Check sheet for the modelled part. Datum: model origin and axes. Units: mm. A direction names the side the tool comes from. Give positions to 0.01 mm unless a question says otherwise; leave off trailing zeros. Loops run counter-clockwise (first coordinate to the right, second up) from the corner with the lowest first, then second, coordinate; pieces in that order, holes last. Notation, with made-up numbers: (86, 84.25) -> (126, 84.25) arc R8 cw to (126, 88.25) -> close; hole circle Ø8 at (31.25, 35). An arc over 180 degrees is marked (long way). Write each question's results on one line, items separated by ' | '. Start each with the question number.
1. Cross-section at A-A on x = -12. Record the boundary of the cut face in (y, z).
2. Mould release check, pull along X, two halves, no side actions. Record for faces 6 (the face through (0, -23, 48)), 7 (the face through (60, -22.5, 24.2)), 8 (the face through (-17.969, -27.137, 46.028)): +X half, -X half, draft (parallel to the pull), parting line (faces both ways), or undercut.
3. Tool access check on faces 1 (the face through (-31, -25, 24)), 2 (the face through (-59.5, 0, 26)), 3 (the face through (26.13, 28.19, 26.38)), 4 (the face through (6, -26, 35)), 5 (the face through (-0.4, -32.5, 44)). Record the directions out of +Z, -Z, +X, -X, +Y, -Y that give a thin tool (end or side, any length) a straight path to the whole face; none if there is none.
4. Cross-section at D-D on x = 41.5. Record the boundary of the cut face in (y, z).
5. Gauge pin test, flat ends, axial feed: pin 1 Ø3.5 at (x, y) = (18, -29) entering from +Z; pin 2 Ø1 at (x, z) = (43, 15.5) entering from +Y; pin 3 Ø2.5 at (y, z) = (-27, 24.5) entering from -X; pin 4 Ø5 at (x, z) = (-28, 20) entering from -Y. Record the tip position at first contact, or that the pin passes through.
6. Material ranges on L1, parallel to Y at x = -17, z = 46; L2, parallel to Y at x = -46.5, z = 26; L3, parallel to X at y = -6, z = 38, recorded low to high. Write a range as from..to.
7. Cross-section at B-B on y = -8. Record the boundary of the cut face in (x, z), and give its area (3 significant figures).
8. Cross-section at C-C on x = 8.5. Record the boundary of the cut face in (y, z), and give its area (3 significant figures).
from build123d import *

# Parameters (mm, degrees)
SKETCH_1_W             = 125
SKETCH_1_H             = 50
EXTRUDE_1_DEPTH        = 3
SKETCH_2_W             = 125
SKETCH_2_H             = 50
SKETCH_2_W_2           = 119
SKETCH_2_H_2           = 44
EXTRUDE_2_DEPTH        = 45
EXTRUDE_START          = 33
EXTRUDE_3_DEPTH        = 12
SKETCH_6_W             = 50
SKETCH_6_H             = 8
SKETCH_6_R             = 2.1
EXTRUDE_7_DEPTH        = 4
FILLET_START           = 43
FILLET_10_DEPTH        = 5
FILLET_START_2         = 44
FILLET_10_2_DEPTH      = 4
CHAMFER_2_SIZE         = 6
FILLET_12_R            = 2
CHAMFER_3_SIZE         = 5
SKETCH_7_R             = 1.35
CUT_EXTRUDE_1_DEPTH    = 86.435648297
PATTERN_LINEAR_2_COUNT = 2
PATTERN_LINEAR_2_PITCH = 39
FILLET_13_R            = 2
SKETCH_8_W             = 12
SKETCH_8_H             = 8
CUT_EXTRUDE_2_DEPTH    = 86.435648297
FILLET_14_R            = 3
SKETCH_9_W             = 61.451933819
SKETCH_9_H             = 10.261376853
CUT_EXTRUDE_3_DEPTH    = 70
SKETCH_10_R            = 3
SKETCH_10_R_2          = 1.5
EXTRUDE_8_DEPTH        = 6.47


with BuildPart() as part:
    # 草图1 → 凸台-拉伸1 (new body)
    with BuildSketch(Plane.XY):
        Rectangle(SKETCH_1_W, SKETCH_1_H)
    extrude(amount=EXTRUDE_1_DEPTH)

    # 草图2 → 凸台-拉伸2 (add)
    with BuildSketch(Plane.XY.offset(3)):
        Rectangle(SKETCH_2_W, SKETCH_2_H)
        Rectangle(SKETCH_2_W_2, SKETCH_2_H_2, mode=Mode.SUBTRACT)
    extrude(amount=EXTRUDE_2_DEPTH)

    # 草图3 → 凸台-拉伸3 (add)
    with BuildSketch(Plane(origin=(0, 0, 0), x_dir=(0, 0, -1), z_dir=(1, 0, 0)).offset(EXTRUDE_START)):
        Polygon((0, 25), (-48, 33), (-48, 25), align=None)
        Polygon((-48, -25), (0, -25), (-48, -33), align=None)
    extrude_3 = extrude(amount=EXTRUDE_3_DEPTH)

    # 草图6 → 凸台-拉伸7 (add)
    # profile 1 of 2: a face of its own
    with BuildSketch(Plane.XY.offset(48)):
        with Locations((0, 29)):
            Rectangle(SKETCH_6_W, SKETCH_6_H)
        with Locations((-17, 29)):
            Circle(SKETCH_6_R, mode=Mode.SUBTRACT)
        with Locations((18, 29)):
            Circle(SKETCH_6_R, mode=Mode.SUBTRACT)
    # profile 2 of 2: a face of its own
    with BuildSketch(Plane.XY.offset(48)):
        with Locations((0, -29)):
            Rectangle(SKETCH_6_W, SKETCH_6_H)
        with Locations(Location((-17, -29, 0), (0, 0, 180))):
            Circle(SKETCH_6_R, mode=Mode.SUBTRACT)
        with Locations((18, -29)):
            Circle(SKETCH_6_R, mode=Mode.SUBTRACT)
    extrude(amount=-EXTRUDE_7_DEPTH)

    # 圆角10: read off the stored shape, not the designer's step
    # 圆角10 outline → 圆角10 (cut)
    with BuildSketch(Plane.XY.offset(FILLET_START)):
        with BuildLine():
            ThreePointArc((25, -29), (23.828427125, -31.828427125), (21, -33))
            Line((21, -33), (25, -33))
            Line((25, -33), (25, -29))
        make_face()
        with BuildLine():
            Line((-25, -33), (-21, -33))
            ThreePointArc((-21, -33), (-23.828427125, -31.828427125), (-25, -29))
            Line((-25, -29), (-25, -33))
        make_face()
        with BuildLine():
            ThreePointArc((-25, 29), (-23.828427125, 31.828427125), (-21, 33))
            Line((-21, 33), (-25, 33))
            Line((-25, 33), (-25, 29))
        make_face()
        with BuildLine():
            Line((25, 33), (21, 33))
            ThreePointArc((21, 33), (23.828427125, 31.828427125), (25, 29))
            Line((25, 29), (25, 33))
        make_face()
    extrude(amount=FILLET_10_DEPTH, mode=Mode.SUBTRACT)

    # Fillet 10 2 outline → Fillet 10 2 (add)
    with BuildSketch(Plane.XY.offset(FILLET_START_2)):
        with BuildLine():
            Line((25, -25), (25, -29))
            ThreePointArc((25, -29), (26.171572875, -26.171572875), (29, -25))
            Line((29, -25), (25, -25))
        make_face()
        with BuildLine():
            ThreePointArc((-29, -25), (-26.171572875, -26.171572875), (-25, -29))
            Line((-25, -29), (-25, -25))
            Line((-25, -25), (-29, -25))
        make_face()
        with BuildLine():
            Line((-25, 25), (-25, 29))
            ThreePointArc((-25, 29), (-26.171572875, 26.171572875), (-29, 25))
            Line((-29, 25), (-25, 25))
        make_face()
        with BuildLine():
            ThreePointArc((29, 25), (26.171572875, 26.171572875), (25, 29))
            Line((25, 29), (25, 25))
            Line((25, 25), (29, 25))
        make_face()
    extrude(amount=FILLET_10_2_DEPTH)

    # 倒角2
    chamfer_2_edges = [part.edges().sort_by_distance(p)[0] for p in [
        (-62.5, 0, 0),
        (62.5, 0, 0),
    ]]
    chamfer(chamfer_2_edges, length=CHAMFER_2_SIZE)

    # 圆角12
    fillet_12_edges = [part.edges().sort_by_distance(p)[0] for p in [
        (0, -22, 3),
        (59.5, 0, 3),
        (0, 22, 3),
        (-59.5, 0, 3),
    ]]
    fillet(fillet_12_edges, radius=FILLET_12_R)

    # 倒角3
    chamfer_3_edges = [part.edges().sort_by_distance(p)[0] for p in [
        (62.5, -25, 27),
        (-62.5, -25, 27),
        (-62.5, 25, 27),
        (62.5, 25, 27),
    ]]
    chamfer(chamfer_3_edges, length=CHAMFER_3_SIZE)

    # 草图7 → 切除-拉伸1 (cut, through all)
    with BuildSketch(Plane(origin=(0, 0, 0), x_dir=(-1, 0, 0), z_dir=(0, 0, -1))):
        with Locations((-12, 0)):
            Circle(SKETCH_7_R)
        with Locations((12, 0)):
            Circle(SKETCH_7_R)
    extrude(amount=-CUT_EXTRUDE_1_DEPTH, mode=Mode.SUBTRACT)

    # 阵列(线性)2: 凸台-拉伸3 ×2
    with Locations(*[(-i * PATTERN_LINEAR_2_PITCH, 0, 0) for i in range(1, PATTERN_LINEAR_2_COUNT)]):
        add(extrude_3)

    # 圆角13
    fillet_13_edges = [part.edges().sort_by_distance(p)[0] for p in [
        (-6, 28.666666667, 22),
        (6, 28.666666667, 22),
        (-6, -28.666666667, 22),
        (6, -28.666666667, 22),
    ]]
    fillet(fillet_13_edges, radius=FILLET_13_R)

    # 草图8 → 切除-拉伸2 (cut, through all)
    with BuildSketch(Plane.XY.offset(48)):
        with Locations((39, 29)):
            Rectangle(SKETCH_8_W, SKETCH_8_H)
        with Locations((39, -29)):
            Rectangle(SKETCH_8_W, SKETCH_8_H)
    extrude(amount=-CUT_EXTRUDE_2_DEPTH, mode=Mode.SUBTRACT)

    # 圆角14
    # the kernel refuses this fillet: 3 mm, written as the material it adds along each edge
    with BuildSketch(Plane(origin=(56.5, 19, 3), x_dir=(0, 1, 0), z_dir=(-1, 0, 0))) as fillet_14_piece_1:
        with BuildLine():
            CenterArc((1, -2), 2, 0, 90)
            Line((3, -2), (3, 0))
            Line((3, 0), (1, 0))
        make_face()
    revolve(axis=Axis((56.5, 19, 3), (0, 0, -1)), revolution_arc=90)
    with BuildSketch(Plane(origin=(56.5, -19, 3), x_dir=(1, 0, 0), z_dir=(0, 1, 0))) as fillet_14_piece_2:
        with BuildLine():
            CenterArc((1, -2), 2, 0, 90)
            Line((3, -2), (3, 0))
            Line((3, 0), (1, 0))
        make_face()
    revolve(axis=Axis((56.5, -19, 3), (0, 0, -1)), revolution_arc=90)
    with BuildSketch(Plane(origin=(-56.5, 19, 3), x_dir=(-1, 0, 0), z_dir=(0, -1, 0))) as fillet_14_piece_3:
        with BuildLine():
            CenterArc((1, -2), 2, 0, 90)
            Line((3, -2), (3, 0))
            Line((3, 0), (1, 0))
        make_face()
    revolve(axis=Axis((-56.5, 19, 3), (0, 0, -1)), revolution_arc=90)
    with BuildSketch(Plane(origin=(-56.5, -19, 3), x_dir=(0, -1, 0), z_dir=(1, 0, 0))) as fillet_14_piece_4:
        with BuildLine():
            CenterArc((1, -2), 2, 0, 90)
            Line((3, -2), (3, 0))
            Line((3, 0), (1, 0))
        make_face()
    revolve(axis=Axis((-56.5, -19, 3), (0, 0, -1)), revolution_arc=90)
    with BuildSketch(Plane(origin=(59.5, -22, 3), x_dir=(0, 1, 0), z_dir=(0, 0, 1))) as fillet_14_piece_5:
        with BuildLine():
            CenterArc((FILLET_14_R, FILLET_14_R), FILLET_14_R, 180, 90)
            Line((0, FILLET_14_R), (0, 0))
            Line((0, 0), (FILLET_14_R, 0))
        make_face()
    extrude(amount=45)
    with BuildSketch(Plane(origin=(59.5, 22, 3), x_dir=(0, -1, 0), z_dir=(0, 0, 1)), Plane(origin=(-59.5, 22, 3), x_dir=(1, 0, 0), z_dir=(0, 0, 1)), Plane(origin=(-59.5, -22, 3), x_dir=(0, 1, 0), z_dir=(0, 0, 1))) as fillet_14_piece_6:
        with BuildLine():
            CenterArc((FILLET_14_R, -FILLET_14_R), FILLET_14_R, 90, 90)
            Line((0, -FILLET_14_R), (0, 0))
            Line((0, 0), (FILLET_14_R, 0))
        make_face()
    extrude(amount=45)

    # 草图9 → 切除-拉伸3 (cut)
    with BuildSketch(Plane(origin=(0, 0, 0), x_dir=(-1, 0, 0), z_dir=(0, 0, -1))):
        with Locations((1.72596691, 30.130688427)):
            Rectangle(SKETCH_9_W, SKETCH_9_H)
    extrude(amount=-CUT_EXTRUDE_3_DEPTH, mode=Mode.SUBTRACT)

    # 草图10 → 凸台-拉伸8 (add)
    # profile 1 of 2: a face of its own
    with BuildSketch(Plane(origin=(0, 25, 0), x_dir=(1, 0, 0), z_dir=(0, 1, 0))):
        with Locations(Location((-29.695093854, -24, 0), (0, 0, 90))):
            Circle(SKETCH_10_R)
        with Locations(Location((-29.695093854, -24, 0), (0, 0, 270))):
            Circle(SKETCH_10_R_2, mode=Mode.SUBTRACT)
    # profile 2 of 2: a face of its own
    with BuildSketch(Plane(origin=(0, 25, 0), x_dir=(1, 0, 0), z_dir=(0, 1, 0))):
        with Locations(Location((24.304906146, -24, 0), (0, 0, 90))):
            Circle(SKETCH_10_R)
        with Locations(Location((24.304906146, -24, 0), (0, 0, 270))):
            Circle(SKETCH_10_R_2, mode=Mode.SUBTRACT)
    extrude(amount=EXTRUDE_8_DEPTH)


solid = part.part
Geometry says:
1) outline: (-33, 44) -> (-25, 44) -> (-25, 0) -> (-1.35, 0) -> (-1.35, 3) -> (-20, 3) arc R2 cw to (-22, 5) -> (-22, 48) -> (-33, 48) -> close; (1.35, 0) -> (25, 0) -> (25, 48) -> (22, 48) -> (22, 5) arc R2 cw to (20, 3) -> (1.35, 3) -> close
2) face 6: draft | face 7: +X half | face 8: undercut
3) face 1: -Z, -X, -Y | face 2: +Z | face 3: +Y | face 4: -Z, +X, -Y | face 5: -Z, -Y
4) outline: (-25, 0) -> (25, 0) -> (25, 48) -> (22, 48) -> (22, 5) arc R2 cw to (20, 3) -> (-20, 3) arc R2 cw to (-22, 5) -> (-22, 48) -> (-25, 48) -> close
5) pin 1: through | pin 2: y = 25 | pin 3: x = -6 | pin 4: y = -25
6) L1: -33..-31.1, -26.9..-22, 22..25 | L2: -25..-22, 22..25 | L3: -62.5..-59.5, 59.5..62.5
7) outline: (-62.5, 6) -> (-56.5, 0) -> (56.5, 0) -> (62.5, 6) -> (62.5, 48) -> (59.5, 48) -> (59.5, 5) arc R2 cw to (57.5, 3) -> (-57.5, 3) arc R2 cw to (-59.5, 5) -> (-59.5, 48) -> (-62.5, 48) -> close | area: 611 mm^2
8) outline: (-33, 44) -> (-25, 44) -> (-25, 0) -> (25, 0) -> (25, 48) -> (22, 48) -> (22, 5) arc R2 cw to (20, 3) -> (-20, 3) arc R2 cw to (-22, 5) -> (-22, 48) -> (-33, 48) -> close | area: 454 mm^2
